The listing builds one solid part. Answer for the finished solid, in the listing's coordinates (mm). Face numbers are marked on the shaded views. A direction names the side the tool comes from. Round coordinates to 2 decimals unless told otherwise and drop trailing zeros. Order: outer loops, then holes, each group sorted by start corner. A loop starts at its lowest first (then second) coordinate and runs counter-clockwise, first axis right, second up. Notation, with made-up numbers: (-21, 54.5) - (-10, 54.5) arc R27 ccw to (-10, 86.5) - close; hole circle Ø8 at (85, -6.5). An arc over 180 degrees is marked (long way). One line per item, written item: value. Start each with the question number.
1. For a pull along Z with two mould halves and no side action, classify the marked faces 1, 2 and 3 as released by +Z, released by -Z, zero draft, split by the parting line, or undercut.
2. Flat-ended cylindrical pins translate along their axes: P1, Ø4, axis at y = -45.5, z = 18.5, coming from the -X side; P2, Ø5, axis at x = -111, y = 53.5, coming from the +Z side; P3, Ø8, axis at y = -73, z = 53, coming from the -X side. Find the tip coordinate at first contact, or state that the pin passes through.
3. Section B-B, the plane z = -28.5 is taken. Give the vertices of the cut face in (x, y).
4. A tool of negligible diameter and unlimited length cuts with its end or side. For the marked faces 4, 5, 6 and 7, from which of +Z, -Z, +X, -X, +Y, -Y can it reach the whole face along a straight path? Write none if from no direction.
5. Straight lines are drawn through the part: line 1 (X direction, y = -107, z = 92); line 2 (Z direction, x = -154, y = -63); line 3 (Z direction, x = -81, y = -67). For each, find the intervals that lie inside material, in ascending order.
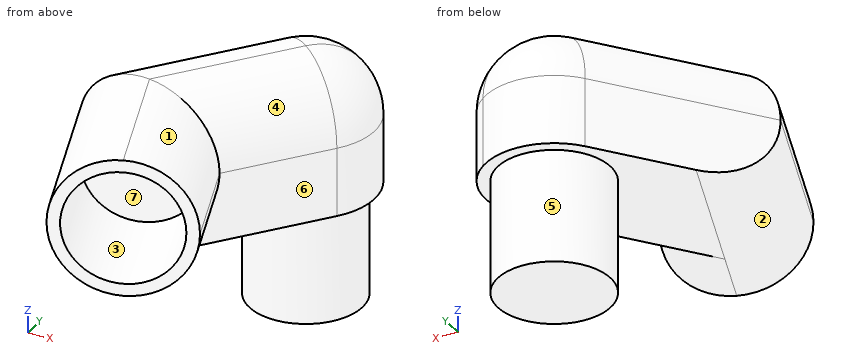
from build123d import *

# Parameters (mm, degrees)
BOSS_EXTRUDE1_DEPTH = 123.444
FILLET1_R           = 61.722
FILLET2_R           = 61.722
SKETCH3_R           = 50.800000000000004
BOSS_EXTRUDE2_DEPTH = 101.6
SKETCH4_R           = 50.8
CUT_EXTRUDE1_DEPTH  = 101.6


with BuildPart() as part:
    # Sketch1 → Boss-Extrude1 (new body)
    with BuildSketch(Plane.XY):
        Polygon((-61.2603734439835, -19.761410788381728), (38.88466731371064, 109.25427234990879), (-58.62951931958517, 184.9471025337958), (-200.27811700244362, 2.4628730865096857), (-144.02441960258417, -155.04747963309688), (-27.772031067671065, -113.52876944205649), align=None)
    extrude(amount=BOSS_EXTRUDE1_DEPTH)

    # Fillet1
    fillet1_edges = [part.edges().sort_by_distance(p)[0] for p in [
        (-44.51620225582728, -66.6450901152191, 123.444),
        (-172.1512683025139, -76.2923032732936, 123.444),
        (-172.1512683025139, -76.2923032732936, 0),
        (-44.51620225582728, -66.6450901152191, 0),
        (-11.187853065136423, 44.74643078076353, 123.444),
        (-129.4538181610144, 93.70498781015274, 123.444),
    ]]
    fillet(fillet1_edges, radius=FILLET1_R - 0.0001)  # a hair under: the kernel refuses the full size

    # Fillet2
    fillet2_edges = [part.edges().sort_by_distance(p)[0] for p in [
        (-58.62951931958517, 184.9471025337958, 30.861050000000017),
        (38.88466731371064, 109.25427234990879, 30.86105000000001),
        (24.604068449214424, 120.33921272724501, 105.36607403771798),
        (-44.34892045508896, 173.86216215645953, 105.366074037718),
    ]]
    fillet(fillet2_edges, radius=FILLET2_R - 0.0001)  # a hair under: the kernel refuses the full size

    # Sketch3 → Boss-Extrude2 (add)
    with BuildSketch(Plane(origin=(0, 0, 0), x_dir=(-1, 0, 0), z_dir=(0, 0, -1))):
        with Locations(Location((47.71884109488077, 98.3435941252044, 0), (0, 0, 180))):
            Circle(SKETCH3_R)
    extrude(amount=BOSS_EXTRUDE2_DEPTH)

    # Sketch4 → Cut-Extrude1 (cut)
    with BuildSketch(Plane(origin=(32.81770626358453, -91.88957753803668, 0), x_dir=(0.9417419115948374, 0.3363363969981563, 0), z_dir=(0.3363363969981563, -0.9417419115948374, 0))):
        with Locations((-126.05994289631548, 61.722)):
            Circle(SKETCH4_R)
    extrude(amount=-CUT_EXTRUDE1_DEPTH, mode=Mode.SUBTRACT)


solid = part.part
Answer list:
1. face 1: released by +Z
1. face 2: released by -Z
1. face 3: undercut
2. P1: stops at x = -166.52
2. P2: stops at z = 120.12
2. P3: stops at x = -174.2
3. outline: circle Ø101.6 at (-47.72, 98.34)
4. face 4: +Z, +X
4. face 5: -Z
4. face 6: -Z, +X
4. face 7: none
5. line 1: x = -152.76 to -138.96, -52.33 to -38.53
5. line 2: z = 14.85 to 30.61, 92.83 to 108.59
5. line 3: z = 6.34 to 18.85, 104.6 to 117.11
